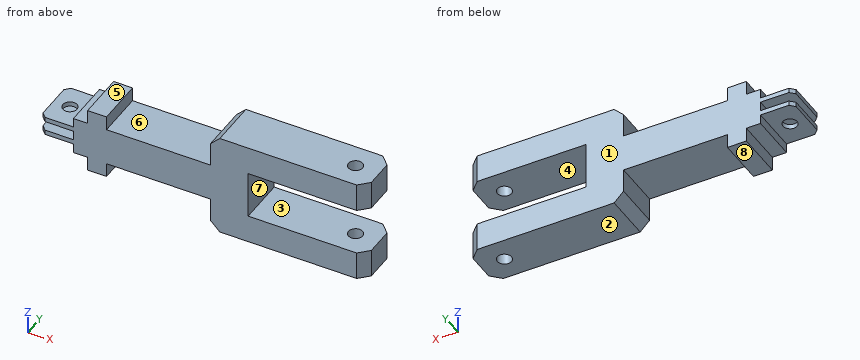
Autodesk Inventor part; units mm, degrees
ref_plane "Work Plane1" through (0, 0, -10) normal (0, 0, 1) x (1, 0, 0)
ref_plane "YZ Plane" through (0, 0, 0) normal (1, 0, 0) x (0, 1, 0)
ref_plane "XZ Plane" through (0, 0, 0) normal (0, 1, 0) x (-1, 0, 0)
ref_plane "Work Plane1" through (0, 0, -10) normal (0, 0, 1) x (1, 0, 0)
sketch "Sketch12" plane through (0, 0, 0) normal (0, 1, 0) x (-1, 0, 0)
  line L0 (5, 4) -> (2, 4)
  line L1 (-2, 4) -> (-2, 7)
  line L2 (-2, 7) -> (2, 7)
  line L3 (2, 7) -> (2, 4)
  line L4 (6, 1) -> (12, 1)
  line L5 (12, -1) -> (6, -1)
  line L6 (12, -1) -> (6, -1)
  line L7 (6, -2) -> (12, -2)
  line L8 (5, -4) -> (5, 4)
  line L9 (12, -2) -> (12, -1)
  line L10 (12, 1) -> (12, 2)
  line L11 (12, 2) -> (6, 2)
  line L12 (6, -2) -> (5, -2)
  line L13 (6, -1) -> (5, -1)
  line L14 (6, 1) -> (5, 1)
  line L15 (6, 2) -> (5, 2)
  line L16 (-31, -11) -> (-57, -11)
  line L17 (-57, -11) -> (-57, -5)
  line L18 (-31, 11) -> (-57, 11)
  line L19 (-57, 11) -> (-57, 5)
  line L20 (-31, -11) -> (-24, -11)
  line L21 (-24, -11) -> (-24, -4)
  line L22 (-24, -4) -> (-24, 11)
  line L23 (-24, 11) -> (-31, 11)
  line L24 (-32, -4) -> (-32, 4)
  line L25 (-32, 4) -> (-32, 5)
  line L26 (-32, 5) -> (-57, 5)
  line L27 (-32, -4) -> (-32, -5)
  line L28 (-32, -5) -> (-57, -5)
  line L29 (5, -4) -> (2, -4)
  line L30 (2, -4) -> (2, -7)
  line L31 (2, -7) -> (-2, -7)
  line L32 (-2, -7) -> (-2, -4)
  line L33 (-2, -4) -> (-5, -4)
  line L34 (-5, -4) -> (-5, 4)
  line L35 (-5, 4) -> (-2, 4)
  line L36 (-5, 4) -> (-24, 4)
  line L37 (-5, -4) -> (-24, -4)
  point P0 (0, 0)
  point P1 (-31, 4)
  dimension "d118" = 4
  dimension "d156" = 7
  dimension "d170" = 3
  dimension "d171" = 3
ref_plane "Work Plane3" through (-12, 0, 2) normal (0, 0, 1) x (1, 0, 0)
extrude "Extrusion16" add sketch "Sketch12" along normal mid plane 10
extrude "Extrusion17" add sketch "Sketch12" along normal mid plane 8 contours L15 L11 L10 L4 L14 L8 | L13 L5 L9 L7 L12 L8
sketch "Sketch17" plane through (-12, 4, 2) normal (0, 0, 1) x (1, 0, 0)
  line L0 (7, -9) -> (7, 1)
  line L1 (7, -8) -> (3.5, -8)
  line L2 (0, -8) -> (7, -8)
  circle A0 centre (3.5, -4) radius 1.5
  point P0 (12, -4)
  point P1 (7, 0)
  dimension "d173" = 3
extrude "Extrusion18" cut sketch "Sketch17" against normal through all
extrude "Extrusion19" add sketch "Sketch12" along normal mid plane 6 contours L22 L21 L20 L16 L17 L28 L27 L24 L25 L26 L19 L18 L23
sketch "Sketch18" plane through (57, 3, -11) normal (0, 0, -1) x (-1, 0, 0)
  line L0 (0, -6) -> (0, 0)
  circle A0 centre (5, -3) radius 1.5
  point P0 (57, -3)
  dimension "d162" = 3
extrude "Extrusion20" cut sketch "Sketch18" against normal through all
chamfer "Chamfer12" distance 2 angle 45 6 edges at (57, 5, 8) (57, -5, 8) (57, 5, -8) (57, -5, -8) (24, 0, 11) (24, 0, -11)
chamfer "Chamfer13" distance 1 angle 45 4 edges at (-12, 5, 1.5) (-12, -5, 1.5) (-12, -5, -1.5) (-12, 5, -1.5)
properties part number "finger"
Geometry check sheet. Reference: the model listing, model coordinates, mm. Face numbers are marked on the shaded views. A direction names the side the tool comes from. Give positions to 0.01 mm unless a question says otherwise; leave off trailing zeros. Write each loop counter-clockwise with the first axis right and the second up, starting at its lowest first coordinate (ties: lowest second). Pieces come first, ordered by that corner, then holes. Notation, with made-up numbers: (19.5, 28) -> (76.5, 28) arc R26 ccw to (76.5, 52) -> close; hole circle Ø10 at (28.25, 6). An arc over 180 degrees is marked (long way). One line per question, with ' | ' between items.
Item 1: Scan lines: line 1 along Y through (x, z) = (52, 6.25); line 2 along Z through (x, y) = (35, 3.5); line 3 along Z through (x, y) = (-7, 1). Record each from-to range of solid material in increasing order.
Determined:
line 1: -5 to -1.5, 1.5 to 5 | line 2: -11 to -5, 5 to 11 | line 3: -2 to -1, 1 to 2
Item 2: Sectioned sample at C-C, the plane z = -3. Record the boundary of the cut face in (x, y), plus the area to 3 significant figures.
Determined:
outline: (-5, -5) -> (32, -5) -> (32, 5) -> (-5, 5) -> close | area: 370 mm^2
Item 3: Depth check by flat-ended pin: pin 1 (5.5 mm diameter, centred on y = 0.5, z = -6.5, fed in from -X); pin 2 (1.5 mm diameter, centred on y = -0.5, z = 6.5, fed in from -X); pin 3 (5.5 mm diameter, centred on x = -9, y = 2, fed in from -Z); pin 4 (2.5 mm diameter, centred on x = 52, y = 0, fed in from +Z). Enter the tip coordinate at first touch or a pass-through.
Determined:
pin 1: x = -5 | pin 2: x = -2 | pin 3: z = -2 | pin 4: through
Item 4: Access from +Z, -Z, +X, -X, +Y, -Y to the whole of each face (thin tool, end or side, straight path). Record for the marked faces 5, 6, 7 and 8.
Determined:
face 5: +Z, -X, +Y, -Y | face 6: +Z, +Y, -Y | face 7: +X, +Y, -Y | face 8: -Z, -X, +Y, -Y
Item 5: Sectioned sample at B-B, the plane x = 33. Record the boundary of the cut face in (y, z), plus the area to 3 significant figures.
Determined:
outline: (-5, -11) -> (5, -11) -> (5, -5) -> (-5, -5) -> close; (-5, 5) -> (5, 5) -> (5, 11) -> (-5, 11) -> close | area: 120 mm^2
Item 6: Sectioned sample at D-D, the plane y = 0. State how many separate pieces and enclosed holes the cut face has, plus the area to 3 significant figures.
Determined:
separate pieces: 5 | enclosed holes: 0 | area: 700 mm^2
Item 7: Draft check along Z on the marked faces 1, 2, 3 and 4. Enter one of: released by +Z, released by -Z, zero draft, split by the parting line, or undercut.
Determined:
face 1: zero draft | face 2: released by -Z | face 3: undercut | face 4: undercut
Item 8: Sectioned sample at A-A, the plane x = 52. Record the boundary of the cut face in (y, z).
Determined:
outline: (-5, -11) -> (-1.5, -11) -> (-1.5, -5) -> (-5, -5) -> close; (-5, 5) -> (-1.5, 5) -> (-1.5, 11) -> (-5, 11) -> close; (1.5, -11) -> (5, -11) -> (5, -5) -> (1.5, -5) -> close; (1.5, 5) -> (5, 5) -> (5, 11) -> (1.5, 11) -> close
